Can you work these out from the model? Positions are in its coordinate system, mm. Face numbers are marked on the shaded views. A direction names the side the tool comes from. Give positions to 0.01 mm unless a question says otherwise; leave off trailing zeros. Write each loop counter-clockwise with the first axis right and the second up, starting at its lowest first coordinate (ties: lowest second). Pieces come first, ordered by that corner, then holes.
1. Suppose I cut it at C-C (x = 139). Please give me the cut outline in (y, z).
2. On a 3-axis mill with a long thin cutter (end or side, diameter ignored), from which of +Z, -Z, +X, -X, +Y, -Y can I reach the whole of each face in a straight line? I mean the marked faces 5 and 6. Say none if no direction works.
3. Suppose I cut it at A-A (y = 0). Please give me the cut outline in (x, z).
4. I'm going to push flat-ended pins straight in: pin 1 (3 mm diameter, centred on x = 12.5, z = -1, fed in from -Y); pin 2 (5 mm diameter, centred on x = 101.5, z = 34, fed in from -Y); pin 3 (8 mm diameter, centred on y = 22, z = 18.5, fed in from +X). Where does each tip first touch, or does it pass through?
5. Thinking about a two-plate mould opening in Y: for the marked faces 1, 2, 3 and 4, which applies, pulls with the +Y half, pulls with the -Y half, needs draft (parallel to the pull), parting line crosses it, or undercut?
6. Suppose I cut it at B-B (x = 80.5). Please give me the cut outline in (y, z).
7. If I drill on probe 1 along X at (y, z) = (7, 23); probe 2 along Y at (x, z) = (33.5, 24); probe 3 along Y at (x, z) = (155, 13), over which ranges is the centre line in solid material (lowest first)?
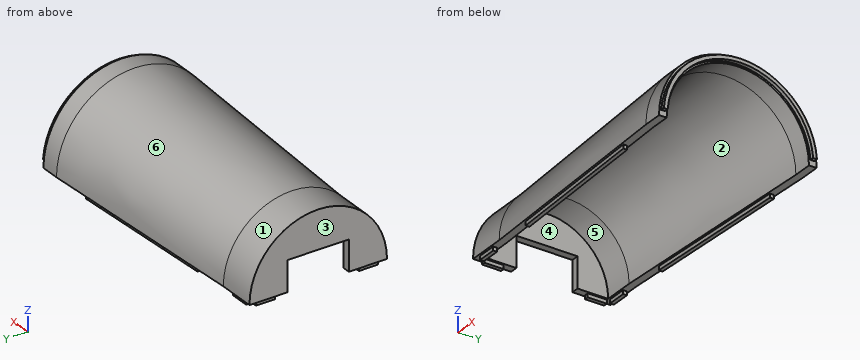
```python
from build123d import *

# Parameters (mm, degrees)
REVOLVE2_ANGLE      = 180
SKETCH4_W           = 20.32
SKETCH4_H           = 20.32
CUT_EXTRUDE2_DEPTH  = 32.004
SKETCH5_W           = 2.54
SKETCH5_H           = 12.7
SKETCH5_W_2         = 12.7
SKETCH5_H_2         = 2.54
BOSS_EXTRUDE1_DEPTH = 2.54
BOSS_EXTRUDE2_DEPTH = 2.54


with BuildPart() as part:
    # Sketch2 → Revolve2 (revolve)
    with BuildSketch(Plane.XY):
        Polygon((0, 0), (0, 40.64), (0, 45.72), (25.4, 45.72), (177.8, 52.373927699), (190.5, 52.373927699), (190.5, 47.293927699), (177.8, 47.293927699), (25.4, 40.64), (5.08, 40.64), (5.08, 0), align=None)
    revolve(axis=Axis((0, 0, 0), (1, 0, 0)), revolution_arc=REVOLVE2_ANGLE)

    # Sketch4 → Cut-Extrude2 (cut)
    with BuildSketch(Plane.ZY):
        with Locations((10.16, 10.16)):
            Rectangle(SKETCH4_W, SKETCH4_H)
        with Locations((10.16, -10.16)):
            Rectangle(SKETCH4_W, SKETCH4_H)
    extrude(amount=-CUT_EXTRUDE2_DEPTH, mode=Mode.SUBTRACT)

    # Sketch5 → Boss-Extrude1 (add)
    with BuildSketch(Plane(origin=(0, 0, 0), x_dir=(-1, 0, 0), z_dir=(0, 0, -1))):
        with Locations((-2.54, 34.29)):
            Rectangle(SKETCH5_W, SKETCH5_H)
        Polygon((-152.4, 49.994939749), (-152.4, 47.454939749), (-50.8, 43.01898795), (-50.8, 45.55898795), align=None)
        with Locations((-11.43, 43.18)):
            Rectangle(SKETCH5_W_2, SKETCH5_H_2)
        Polygon((-50.8, -43.01898795), (-50.8, -45.55898795), (-152.4, -49.994939749), (-152.4, -47.454939749), align=None)
        with Locations((-11.43, -43.18)):
            Rectangle(SKETCH5_W_2, SKETCH5_H_2)
        with Locations((-2.54, -34.29)):
            Rectangle(SKETCH5_W, SKETCH5_H)
    extrude(amount=BOSS_EXTRUDE1_DEPTH)

    # Sketch6 → Boss-Extrude2 (add)
    with BuildSketch(Plane(origin=(190.5, 0, 0), x_dir=(0, 0, -1), z_dir=(1, 0, 0))):
        with BuildLine():
            Line((-3.81, 50.911637334), (-3.81, 48.371637334))
            ThreePointArc((-3.81, 48.371637334), (-48.52145297, 0), (-3.81, -48.371637334))
            Line((-3.81, -48.371637334), (-3.81, -50.911637334))
            ThreePointArc((-3.81, -50.911637334), (-51.054, 0), (-3.81, 50.911637334))
        make_face()
    extrude(amount=BOSS_EXTRUDE2_DEPTH)


solid = part.part
```
Checks:
1. outline: (-50.68, 0) - (-49.41, 0) - (-49.41, -2.54) - (-46.87, -2.54) - (-46.87, 0) - (-45.6, 0) arc R45.6 cw to (45.6, 0) - (46.87, 0) - (46.87, -2.54) - (49.41, -2.54) - (49.41, 0) - (50.68, 0) arc R50.68 ccw to start
2. face 5: -Z, +X
2. face 6: +Z, -X
3. outline: (0, 20.32) - (5.08, 20.32) - (5.08, 40.64) - (25.4, 40.64) - (177.8, 47.29) - (190.5, 47.29) - (190.5, 48.52) - (193.04, 48.52) - (193.04, 51.05) - (190.5, 51.05) - (190.5, 52.37) - (177.8, 52.37) - (25.4, 45.72) - (0, 45.72) - close
4. pin 1: stops at y = -45.72
4. pin 2: stops at y = -37.59
4. pin 3: stops at x = 5.08
5. face 1: parting line crosses it
5. face 2: undercut
5. face 3: needs draft
5. face 4: undercut
6. outline: (-48.13, 0) - (-46.86, 0) - (-46.86, -2.54) - (-44.32, -2.54) - (-44.32, 0) - (-43.05, 0) arc R43.05 cw to (43.05, 0) - (44.32, 0) - (44.32, -2.54) - (46.86, -2.54) - (46.86, 0) - (48.13, 0) arc R48.13 ccw to start
7. probe 1: x = 0 to 5.08
7. probe 2: y = -39.33 to -33.23, 33.23 to 39.33
7. probe 3: y = -49.71 to -44.44, 44.44 to 49.71
